Work out the finished part from the listing and answer in its coordinate system (mm). Face numbers are marked on the shaded views. A direction names the side the tool comes from. Coordinates: 2 decimals unless noted, no trailing zeros. Write each loop counter-clockwise with the first axis right and the second up, starting at its lowest first coordinate (ties: lowest second). Pieces come first, ordered by that corner, then holes. Notation, with made-up numbers: M -11.5,84.5 L 1.5,84.5 A23 cw 1.5,114.5 Z; hole C 48.5,-36.75 d3. An arc over 180 degrees is marked long. Answer as CSV lines item,"result". Start each with the question number.
(1) Find the intervals of material crossed by L1, parallel to Z at x = -2, y = -70; L2, parallel to X at y = 155, z = 2; L3, parallel to Y at x = -15.5, z = 2.5, in increasing order. Write a range as [from, to].
(2) Flat-ended cylindrical pins translate along their axes: P1, Ø5, axis at y = -32.5, z = 23, coming from the +X side; P2, Ø5, axis at y = -27.5, z = 28, coming from the -X side; P3, Ø1, axis at x = -32.5, y = -92.5, coming from the +Z side. Find the tip coordinate at first contact, or state that the pin passes through.
(3) A cutting plane is placed at C-C on z = 31.5. Give the vertices of the cut face in (x, y).
(4) For the marked faces 1 and 2, determine the directions among +Z, -Z, +X, -X, +Y, -Y from which every point of the face is accessible in a straight line to the end or side of a thin tool.
(5) A cutting plane is placed at B-B on y = 60.5. Give the vertices of the cut face in (x, z).
(6) A cutting plane is placed at A-A on x = -32. Give the vertices of the cut face in (y, z).
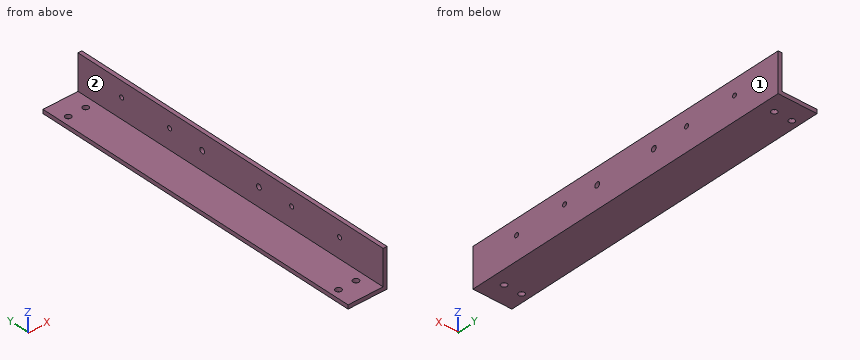
Solid Edge part; units mm, degrees
sketch "Sketch1" plane through (-9.04, 0, 33.0648) normal (0, -1, 0) x (1, 0, 0)
  line L0 (-30.96, -29.0648) -> (5.04, -29.0648)
  line L1 (5.04, -29.0648) -> (5.04, 6.9352)
  line L2 (5.04, 6.9352) -> (9.04, 6.9352)
  line L3 (9.04, 6.9352) -> (9.04, -33.0648)
  line L4 (9.04, -33.0648) -> (-30.96, -33.0648)
  line L5 (-30.96, -33.0648) -> (-30.96, -29.0648)
extrude "Protrusion1" add sketch "Sketch1" along normal mid plane 350
sketch "Sketch2" plane through (-20, 0, 0) normal (0, 0, -1) x (0, -1, 0)
  circle A0 centre (-155, 12) radius 3
  circle A1 centre (-155, -6) radius 3
  dimension "D1" = 155
  dimension "D2" = 155
extrude "Cutout1" cut sketch "Sketch2" against normal through all
mirror "Mirror1" about plane through (0, 0, 0) normal (0, -1, 0) of "Cutout1"
sketch "Sketch3" plane through (0, 0, 20) normal (1, 0, 0) x (0, -1, 0)
  circle A0 centre (-32.5, -3) radius 2.75
  circle A1 centre (32.5, -3) radius 2.75
  dimension "D1" = 32.5
extrude "Cutout2" cut sketch "Sketch3" against normal through all
sketch "Sketch4" plane through (0, 0, 20) normal (1, 0, 0) x (0, -1, 0)
  circle A0 centre (70, -4.37) radius 2.25
  circle A1 centre (125, -4.37) radius 2.25
extrude "Cutout3" cut sketch "Sketch4" against normal through all
mirror "Mirror2" about plane through (0, 0, 0) normal (0, -1, 0) of "Cutout3"
Here are the results:
1,L1,"z = [0, 22.12], [26.62, 40]"
1,L2,"x = [-40, -35], [-29, -17], [-11, 0]"
1,L3,"y = [-175, -157.6], [-152.4, 152.4], [157.6, 175]"
2,P1,"passes through"
2,P2,"stops at x = -4"
2,P3,"stops at z = 4"
3,outline,"M -4,-175 L 0,-175 L 0,175 L -4,175 Z"
4,face 1,"+Z, -Z, +X, +Y, -Y"
4,face 2,"+Z, -X, +Y, -Y"
5,outline,"M -40,0 L 0,0 L 0,40 L -4,40 L -4,4 L -40,4 Z"
6,outline,"M -175,0 L -158,0 L -158,4 L -175,4 Z; M -152,0 L 152,0 L 152,4 L -152,4 Z; M 158,0 L 175,0 L 175,4 L 158,4 Z"
